Geometry: final body of the model. Coordinates: model frame, mm. Face numbers are marked on the shaded views. A direction names the side the tool comes from. Coordinates: 2 decimals unless noted, no trailing zeros. Order: outer loops, then holes, each group sorted by start corner. A loop starts at its lowest first (then second) coordinate and runs counter-clockwise, first axis right, second up. Notation, with made-up numbers: (58, -7.75) -> (77, -7.75) arc R24 ccw to (77, 18.25) -> close; hole circle Ø5 at (50.25, 3). An arc over 180 degrees is marked (long way). Answer in a Markdown table with one row per item. Add a question column.
1) Set-up query: the marked faces 1 and 2. Return all of +Z, -Z, +X, -X, +Y, -Y with unobstructed straight access to the full face (end or side cutting, diameter ignored); none if empty.
2) Section query A-A on z = -10. Return the cut outline in (x, y).
3) Ray query, line 1 (Z direction, x = -2.5, y = 10.5); line 2 (X direction, y = -9.5, z = 55.5); line 3 (Z direction, x = -12, y = -2). Return the intervals inside material, ascending. Write a range as from..to.
4) Contact query for flat-ended pins moving along their axis: P1, Ø10, axis at y = -5, z = 0.5, coming from the -X side; P2, Ø8, axis at x = -2, z = 46.5, coming from the -Y side; P3, Ø1.5, axis at x = 11.5, z = 6, coming from the +Y side; P4, Ø3, axis at x = -9, z = -5, coming from the +Y side. Output: stop coordinate, or through.
```python
from build123d import *

# Parameters (mm, degrees)
F2_R     = 6.35
F3_DEPTH = 19.05


with BuildPart() as f1:
    # F0 (on Front) → F1 (revolve)
    with BuildSketch(Plane.XZ):
        with BuildLine():
            Line((-14.2875, 0), (0, 0))
            Line((0, 0), (0, 82.55))
            add(Edge.make_bspline(
                [(-10.3173267766, 13.7772673566), (-9.7542577342, 13.9189949448), (-8.7837192186, 14.0342974796), (-6.7366964189, 15.6271610186), (-5.7831889647, 17.2510746377), (-5.3274903025, 19.561240103), (-6.3597783763, 21.6465588891), (-7.8655763238, 23.5184731931), (-11.4427663168, 24.8942017837), (-15.9643108763, 28.067693587), (-19.0623897098, 34.6572420873), (-20.4563878975, 44.6646724068), (-17.1595032199, 56.3004961078), (-12.3601997394, 67.5904391591), (-3.8765890058, 79.7095969319), (0, 82.55)],
                knots=[0, 0, 0, 0, 0.0415999938, 0.0933658969, 0.139413565, 0.1887556661, 0.2383289481, 0.28858266, 0.352549029, 0.4293674027, 0.5174702969, 0.6222470639, 0.7355863968, 0.8559952045, 1, 1, 1, 1], degree=3))
            Line((-10.3173267766, 13.7772673566), (-10.3173267766, 12.1897673566))
            ThreePointArc((-10.3173267766, 12.1897673566), (-12.0615351158, 10.4464615054), (-12.7, 8.0645))
            Line((-12.7, 8.0645), (-14.2875, 8.0645))
            Line((-14.2875, 8.0645), (-14.2875, 0))
        make_face()
    revolve(axis=Axis((0, 0, 41.275), (0, 0, -1)))

    # F2 (on face) → F3 (join)
    with BuildSketch(Plane(origin=(0, 0, 0), x_dir=(1, 0, 0), z_dir=(0, 0, -1))):
        Circle(F2_R)
    extrude(amount=F3_DEPTH)


solid = f1.part
```
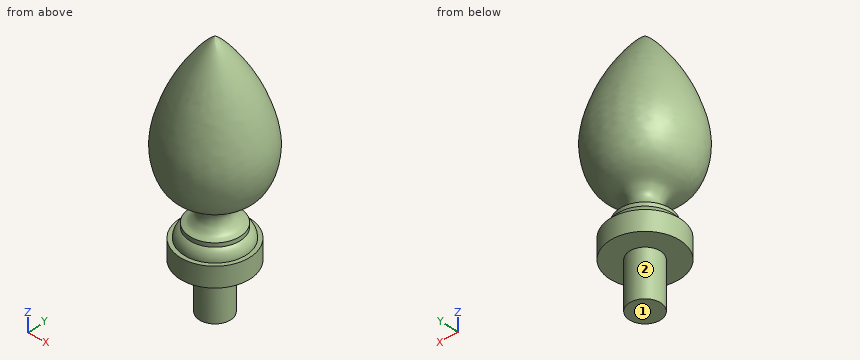
Result:
| question | item | result |
|---|---|---|
| 1 | face 1 | -Z, +X, -X, +Y, -Y |
| 1 | face 2 | -Z |
| 2 | outline | circle Ø12.7 at (0, 0) |
| 3 | line 1 | 0..11.88, 24.77..69.12 |
| 3 | line 2 | -14.31..14.31 |
| 3 | line 3 | 0..10.26, 25.53..66.76 |
| 4 | P1 | x = -14.29 |
| 4 | P2 | y = -19.76 |
| 4 | P3 | y = 9.41 |
| 4 | P4 | through |
